```python
from build123d import *

# Parameters (mm, degrees)
F1_DEPTH = 12.7
F2_ANGLE = 270
F3_W     = 7.3
F3_H     = 12
F4_DEPTH = 7.2
F6_DEPTH = 54.9
F7_R     = 2.8925
F8_DEPTH = 3.5


with BuildPart() as f1:
    # F0 (on Top) → F1 (new body)
    with BuildSketch(Plane.XY):
        Polygon((20.15, 10), (20.15, 0), (20.15, -10), (-20.15, -10), (-20.15, 0), (-20.15, 10), (-27.45, 10), (-27.45, -10), (-27.45, -17.3), (27.45, -17.3), (27.45, -10), (27.45, 10), align=None)
    extrude(amount=F1_DEPTH)


with BuildPart() as f1_1:
    # F2: moved
    add(f1.part.rotate(Axis((0, -17.3, 12.7), (-1, 0, 0)), F2_ANGLE))

    # F3 (on face) → F4 (cut)
    with BuildSketch(Plane.XZ.offset(17.3)):
        with Locations((23.8, 34)):
            Rectangle(F3_W, F3_H)
        with Locations((-23.8, 34)):
            Rectangle(F3_W, F3_H)
    extrude(amount=-F4_DEPTH, mode=Mode.SUBTRACT)

    # F5 (on face) → F6 (cut)
    with BuildSketch(Plane.YZ.offset(27.45)):
        Polygon((-12.3, 40), (-12.3, 28), (-12.3, 20), (-9.6, 20), (-9.6, 40), align=None)
    extrude(amount=-F6_DEPTH, mode=Mode.SUBTRACT)

    # F7 (on face) → F8 (cut)
    with BuildSketch(Plane(origin=(0, 0, 12.7), x_dir=(1, 0, 0), z_dir=(0, 0, -1))):
        with Locations((0, 10.95)):
            Circle(F7_R)
    extrude(amount=-F8_DEPTH, mode=Mode.SUBTRACT)


with BuildPart() as f1_2:
    # F9: moved
    add(f1_1.part.moved(Location((0, 10.95, -12.7))))


solid = f1_2.part
```
Design review of the part built by this model. Coordinates are the model's own, in mm. A direction names the side the tool comes from. Coordinates: 2 decimals unless noted, no trailing zeros. Write each loop counter-clockwise with the first axis right and the second up, starting at its lowest first coordinate (ties: lowest second). Pieces come first, ordered by that corner, then holes.
1) To check wall thickness, follow L1, parallel to X at y = -5.25, z = 7.75; L2, parallel to Y at x = 0, z = 2.1; L3, parallel to X at y = 0, z = 1.5. State the ranges of each line that lie inside material, in increasing order.
2) Add section C-C (z = 14.25). Write out the cut boundary in (x, y), plus the area to 3 significant figures.
3) Add section B-B (y = -3.5). Write out the cut boundary in (x, z).
4) Insertion check: pin 1 (1.5 mm diameter, centred on x = -0.5, y = 0.5, fed in from -Z); pin 2 (6.5 mm diameter, centred on x = 0, y = 0, fed in from +Z); pin 3 (1.5 mm diameter, centred on x = -25, y = -4.5, fed in from +Z). Each pin has a flat end and moves straight along its axis. Give the tip position at first contact, or say it passes through.
5) Add section D-D (x = -23). Write out the cut boundary in (y, z).
6) Machinability: for faces 4 (the flat face through (-24, -1.35, 11)), 5 (the flat face through (20.15, 4, 17)), 6 (the flat face through (-27.45, 2, 11)), 7 (the flat face through (24, -4, 15.3)), which of the approach directions +Z, -Z, +X, -X, +Y, -Y give a long, thin tool a straight path to every point of the face, cutting with its end or side? Answer none if there is none.
7) Mouldability with a two-part tool opening along Y and no side actions: class faces 1 (the flat face through (20.15, -4, 11)), 2 (the flat face through (0, -6.35, 4)), 3 (the cylindrical face through (1.55, -2.44, 1.73)) as +Y half, -Y half, draft (parallel to the pull), parting line (faces both ways), or undercut.
8) Add section A-A (z = 20.75). Write out the cut boundary in (x, y), plus the area to 3 significant figures.
Check result:
1. L1: x = -27.45 to -20.15, 20.15 to 27.45
1. L2: y = -6.35 to -2.89, 2.89 to 6.35
1. L3: x = -27.45 to -2.89, 2.89 to 27.45
2. outline: (-27.45, -6.35) - (-20.15, -6.35) - (-20.15, -1.35) - (-27.45, -1.35) - close; (-27.45, 1.35) - (-20.15, 1.35) - (-20.15, 6.35) - (-27.45, 6.35) - close; (20.15, -6.35) - (27.45, -6.35) - (27.45, -1.35) - (20.15, -1.35) - close; (20.15, 1.35) - (27.45, 1.35) - (27.45, 6.35) - (20.15, 6.35) - close
2. area: 146 mm2
3. outline: (-27.45, 0) - (27.45, 0) - (27.45, 15.3) - (20.15, 15.3) - (20.15, 7.3) - (-20.15, 7.3) - (-20.15, 15.3) - (-27.45, 15.3) - close
4. pin 1: stops at z = 3.5
4. pin 2: stops at z = 7.3
4. pin 3: stops at z = 15.3
5. outline: (-6.35, 0) - (6.35, 0) - (6.35, 27.3) - (1.35, 27.3) - (1.35, 7.3) - (-1.35, 7.3) - (-1.35, 15.3) - (-6.35, 15.3) - close
6. face 4: +Z, +X, -X
6. face 5: +Z, +Y, -Y
6. face 6: +Z, -Z, -X, +Y, -Y
6. face 7: +Z, +X, -X, -Y
7. face 1: draft
7. face 2: -Y half
7. face 3: undercut
8. outline: (-27.45, 1.35) - (-20.15, 1.35) - (-20.15, 6.35) - (-27.45, 6.35) - close; (20.15, 1.35) - (27.45, 1.35) - (27.45, 6.35) - (20.15, 6.35) - close
8. area: 73.0 mm2
